Verification items for this drawing (mm, ordinates from the low corner). A direction names the side the tool comes from. Round coordinates to 2 decimals unless told otherwise and drop trailing zeros. Order: outer loops, then holes, each group sorted by start corner. A loop starts at its lowest first (then second) coordinate and runs counter-clockwise, first axis right, second up. Notation, with made-up numbers: (30, 0) - (45, 0) arc R36 ccw to (45, 37) - close; hole circle Ø1 at (35, 43.25). An arc over 180 degrees is marked (long way). Use a Markdown table: item, result. Add a question column.
(1) Gauge pin test, flat end, axial feed: P1, Ø3, axis at x = 10, y = 10, coming from the +Z side. Record the tip position at first contact, or that the pin passes through.
(2) Thickness scan on line 1 along Y through (x, z) = (10, 5.5); line 2 along X through (y, z) = (17, 9.25); line 3 along Y through (x, z) = (27.75, 9.25). Record the ranges inside material, lowest first. Write a range as [from, to].
(3) Mould release check, pull along Y, two halves, no side actions. Record for the marked faces 3, 4 and 5: released by +Y, released by -Y, zero draft, split by the parting line, or undercut.
(4) Section check B-B on y = 10. Record the boundary of the cut face in (x, z).
(5) Access from +Z, -Z, +X, -X, +Y, -Y to the whole of each face (thin tool, end or side, straight path). Record for the marked faces 1 and 2.
(6) Section check C-C on y = 4. Record the boundary of the cut face in (x, z), then the cut area to 3 significant figures.
(7) Section check D-D on z = 3.75. Give the number of separate pieces and of enclosed holes in the cut face, then the cut area to 3 significant figures.
(8) Section check A-A on x = 10. Record the boundary of the cut face in (y, z), then the cut area to 3 significant figures.
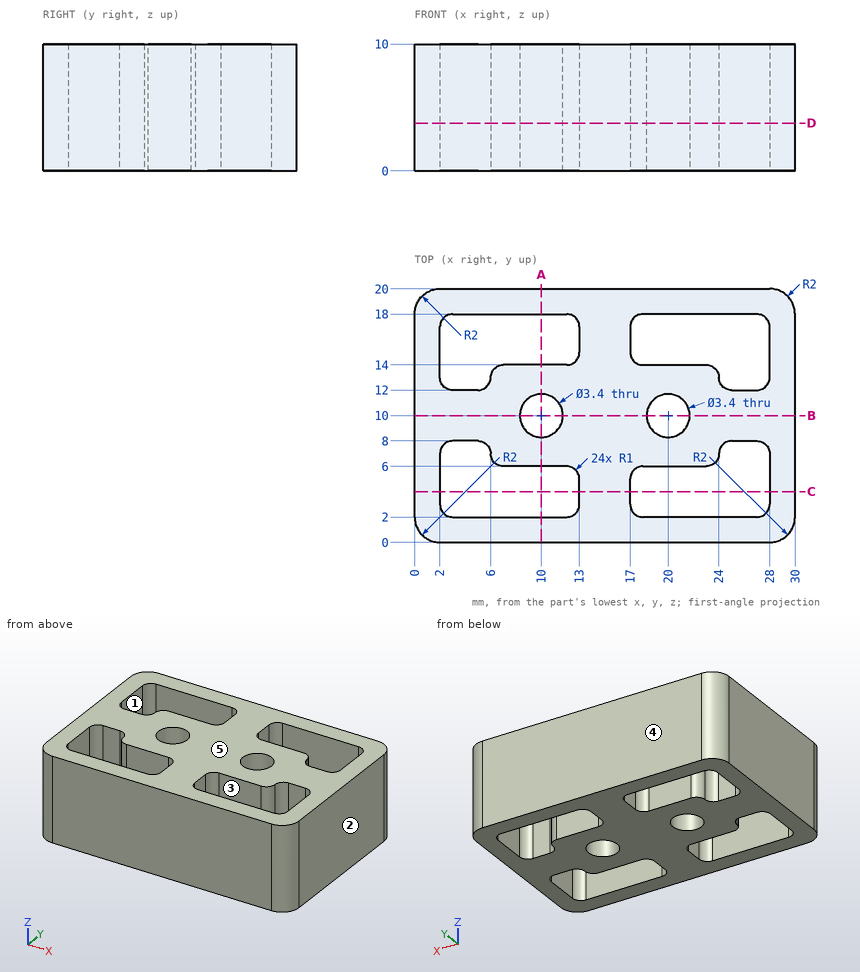
Check sheet entries:
| question | item | result |
|---|---|---|
| 1 | P1 | passes through |
| 2 | line 1 | y = [0, 2], [6, 8.3], [11.7, 14], [18, 20] |
| 2 | line 2 | x = [0, 2], [13, 17], [28, 30] |
| 2 | line 3 | y = [0, 2.34], [7.66, 12.34], [17.66, 20] |
| 3 | face 3 | undercut |
| 3 | face 4 | released by +Y |
| 3 | face 5 | zero draft |
| 4 | outline | (0, 0) - (8.3, 0) - (8.3, 10) - (0, 10) - close; (11.7, 0) - (18.3, 0) - (18.3, 10) - (11.7, 10) - close; (21.7, 0) - (30, 0) - (30, 10) - (21.7, 10) - close |
| 5 | face 1 | +Z, -Z |
| 5 | face 2 | +Z, -Z, +X, +Y, -Y |
| 6 | outline | (0, 0) - (2, 0) - (2, 10) - (0, 10) - close; (13, 0) - (17, 0) - (17, 10) - (13, 10) - close; (28, 0) - (30, 0) - (30, 10) - (28, 10) - close |
| 6 | area | 80.0 mm2 |
| 7 | separate pieces | 1 |
| 7 | enclosed holes | 6 |
| 7 | area | 374 mm2 |
| 8 | outline | (0, 0) - (2, 0) - (2, 10) - (0, 10) - close; (6, 0) - (8.3, 0) - (8.3, 10) - (6, 10) - close; (11.7, 0) - (14, 0) - (14, 10) - (11.7, 10) - close; (18, 0) - (20, 0) - (20, 10) - (18, 10) - close |
| 8 | area | 86.0 mm2 |
